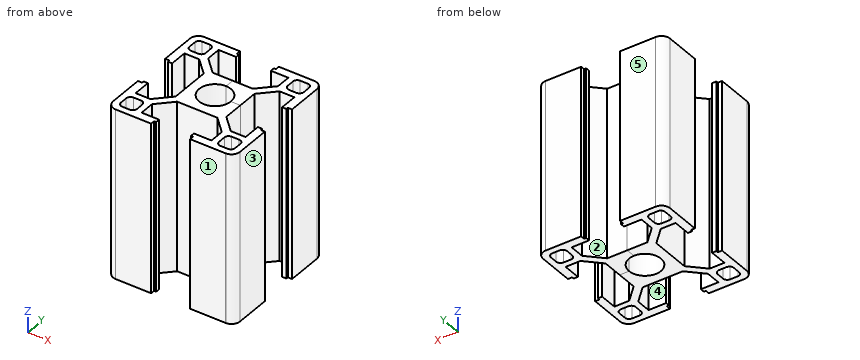
Autodesk Inventor part; units mm, degrees
ref_plane "YZ Plane" through (0, 0, 0) normal (1, 0, 0) x (0, 1, 0)
ref_plane "XZ Plane" through (0, 0, 0) normal (0, 1, 0) x (-1, 0, 0)
ref_plane "XY Plane" through (0, 0, 0) normal (0, 0, 1) x (1, 0, 0)
sketch "Sketch1" plane through (0, 0, 0) normal (0, 0, 1) x (1, 0, 0)
  line L0 (-4.1, 13) -> (-4.1, 14)
  line L1 (-4.1, 14) -> (-4.6, 14)
  line L2 (-4.6, 14) -> (-4.6, 15)
  line L3 (-4.6, 14) -> (-4.6, 15)
  line L4 (-4.6, 15) -> (-13, 15)
  arc A0 (-13, 15) -> (-15, 13) centre (-13, 13) ccw
  line L5 (-15, 13) -> (-15, 4.6)
  line L6 (-15, 13) -> (-15, 4.6)
  line L7 (-15, 4.6) -> (-14, 4.6)
  line L8 (-15, 4.6) -> (-14, 4.6)
  line L9 (-14, 4.6) -> (-14, 4.1)
  line L10 (-14, 4.6) -> (-14, 4.1)
  line L11 (-14, 4.1) -> (-13, 4.1)
  line L12 (-13, 4.1) -> (-13, 8.25)
  line L13 (-13, 8.25) -> (-9.5, 8.25)
  line L14 (-13, 8.25) -> (-9.5, 8.25)
  line L15 (-9.5, 8.25) -> (-6, 4.75)
  line L16 (-6, 4.75) -> (-6, -4.75)
  line L17 (-6, 4.75) -> (-6, -4.75)
  line L18 (-6, -4.75) -> (-9.5, -8.25)
  line L19 (-14, -4.1) -> (-13, -4.1)
  line L20 (-13, -4.1) -> (-14, -4.1)
  line L21 (-14, -4.6) -> (-14, -4.1)
  line L22 (-14, -4.1) -> (-14, -4.6)
  line L23 (-15, -4.6) -> (-14, -4.6)
  line L24 (-14, -4.6) -> (-15, -4.6)
  line L25 (-8.25, 13) -> (-4.1, 13)
  line L26 (-4.1, 13) -> (-8.25, 13)
  line L27 (-8.25, 9.5) -> (-8.25, 13)
  line L28 (-8.25, 13) -> (-8.25, 9.5)
  line L29 (-4.75, 6) -> (-8.25, 9.5)
  line L30 (-8.25, 9.5) -> (-4.75, 6)
  line L31 (4.75, 6) -> (-4.75, 6)
  line L32 (-4.75, 6) -> (4.75, 6)
  line L33 (4.75, 6) -> (8.25, 9.5)
  line L34 (8.25, 13) -> (8.25, 9.5)
  line L35 (8.25, 9.5) -> (8.25, 13)
  line L36 (8.25, 13) -> (4.1, 13)
  line L37 (4.1, 13) -> (4.1, 14)
  line L38 (4.6, 14) -> (4.1, 14)
  line L39 (4.1, 14) -> (4.6, 14)
  line L40 (4.6, 15) -> (4.6, 14)
  line L41 (4.6, 14) -> (4.6, 15)
  line L42 (4.6, 15) -> (13.08, 15)
  line L43 (15, 4.6) -> (15, 13)
  line L44 (15, 13) -> (15, 4.6)
  line L45 (14, 4.6) -> (15, 4.6)
  line L46 (15, 4.6) -> (14, 4.6)
  line L47 (14, 4.6) -> (14, 4.1)
  line L48 (13, 4.1) -> (14, 4.1)
  line L49 (14, 4.1) -> (13, 4.1)
  line L50 (13, 4.1) -> (13, 8.25)
  line L51 (9.5, 8.25) -> (13, 8.25)
  line L52 (13, 8.25) -> (9.5, 8.25)
  line L53 (6, 4.75) -> (9.5, 8.25)
  line L54 (9.5, 8.25) -> (6, 4.75)
  line L55 (6, 4.75) -> (6, -4.75)
  circle A1 centre (0, 0) radius 3.75
  line L56 (0, 0) -> (7.2487, 0)
  arc A2 (15, 13) -> (13, 15) centre (13, 13) ccw
  arc A3 (15, 13) -> (13.08, 15) centre (12.9977, 12.9994) ccw
  line L57 (-9.5, -8.25) -> (-6, -4.75)
  line L58 (-8.25, -9.5) -> (-4.75, -6)
  line L59 (-4.75, -6) -> (-8.25, -9.5)
  line L60 (-4.1, -13) -> (-4.1, -14)
  line L61 (-4.1, -14) -> (-4.6, -14)
  line L62 (-8.25, -13) -> (-4.1, -13)
  line L63 (-4.1, -13) -> (-8.25, -13)
  line L64 (-8.25, -9.5) -> (-8.25, -13)
  line L65 (-8.25, -13) -> (-8.25, -9.5)
  line L66 (-13, -8.25) -> (-9.5, -8.25)
  line L67 (-13, -4.1) -> (-13, -8.25)
  line L68 (-4.6, -14) -> (-4.6, -15)
  line L69 (-4.6, -14) -> (-4.6, -15)
  line L70 (-4.6, -15) -> (-13, -15)
  line L71 (-14, -4.6) -> (-14, -4.1)
  line L72 (-14, -4.6) -> (-14, -4.1)
  line L73 (-14, -4.1) -> (-13, -4.1)
  line L74 (-15, -4.6) -> (-14, -4.6)
  line L75 (-15, -4.6) -> (-14, -4.6)
  line L76 (-15, -13) -> (-15, -4.6)
  line L77 (-15, -13) -> (-15, -4.6)
  arc A4 (-15, -13) -> (-13, -15) centre (-13, -13) ccw
  line L78 (-13, -8.25) -> (-9.5, -8.25)
  line L79 (8.25, -13) -> (8.25, -9.5)
  line L80 (8.25, -9.5) -> (8.25, -13)
  line L81 (9.5, -8.25) -> (13, -8.25)
  line L82 (13, -8.25) -> (9.5, -8.25)
  line L83 (15, -13) -> (15, -4.6)
  line L84 (15, -4.6) -> (15, -13)
  line L85 (13, -4.1) -> (13, -8.25)
  line L86 (13, -4.1) -> (14, -4.1)
  line L87 (14, -4.1) -> (13, -4.1)
  line L88 (14, -4.6) -> (14, -4.1)
  line L89 (14, -4.6) -> (15, -4.6)
  line L90 (15, -4.6) -> (14, -4.6)
  line L91 (4.75, -6) -> (8.25, -9.5)
  line L92 (6, -4.75) -> (9.5, -8.25)
  line L93 (9.5, -8.25) -> (6, -4.75)
  arc A5 (13, -15) -> (15, -13) centre (13, -13) ccw
  arc A6 (13.08, -15) -> (15, -13) centre (12.9977, -12.9994) ccw
  line L94 (8.25, -13) -> (4.1, -13)
  line L95 (4.1, -13) -> (4.1, -14)
  line L96 (4.6, -14) -> (4.1, -14)
  line L97 (4.1, -14) -> (4.6, -14)
  line L98 (4.6, -15) -> (4.6, -14)
  line L99 (4.6, -14) -> (4.6, -15)
  line L100 (4.6, -15) -> (13.08, -15)
  line L101 (4.75, -6) -> (-4.75, -6)
  line L102 (-4.75, -6) -> (4.75, -6)
  circle A7 centre (0, 0) radius 3.75
  line L103 (-12.5, 13.5) -> (-10.7, 13.5)
  line L104 (-12.5, 13.5) -> (-10.7, 13.5)
  line L105 (-9.7, 12.5) -> (-9.7, 10.7)
  line L106 (-9.7, 12.5) -> (-9.7, 10.7)
  line L107 (-10.7, 9.7) -> (-12.5, 9.7)
  line L108 (-10.7, 9.7) -> (-12.5, 9.7)
  line L109 (-13.5, 12.5) -> (-13.5, 10.7)
  line L110 (-13.5, 10.7) -> (-13.5, 12.5)
  line L111 (-13.5, 12.5) -> (-13.5, 10.7)
  arc A8 (-12.5, 13.5) -> (-13.5, 12.5) centre (-12.5, 12.5) ccw
  arc A9 (-13.5, 10.7) -> (-12.5, 9.7) centre (-12.5, 10.7) ccw
  arc A10 (-13.5, 10.7) -> (-12.5, 9.7) centre (-12.5, 10.7) ccw
  arc A11 (-10.7, 9.7) -> (-9.7, 10.7) centre (-10.7, 10.7) ccw
  arc A12 (-9.7, 12.5) -> (-10.7, 13.5) centre (-10.7, 12.5) ccw
  arc A13 (-9.7, 12.5) -> (-10.7, 13.5) centre (-10.7, 12.5) ccw
  line L112 (0, 0) -> (0, 6.5)
  arc A14 (9.7, 10.7) -> (10.7, 9.7) centre (10.7, 10.7) ccw
  line L113 (9.7, 12.5) -> (9.7, 10.7)
  arc A15 (10.7, 13.5) -> (9.7, 12.5) centre (10.7, 12.5) ccw
  arc A16 (10.7, 13.5) -> (9.7, 12.5) centre (10.7, 12.5) ccw
  line L114 (9.7, 12.5) -> (9.7, 10.7)
  line L115 (12.5, 13.5) -> (10.7, 13.5)
  line L116 (12.5, 13.5) -> (10.7, 13.5)
  line L117 (10.7, 9.7) -> (12.5, 9.7)
  line L118 (10.7, 9.7) -> (12.5, 9.7)
  arc A17 (12.5, 9.7) -> (13.5, 10.7) centre (12.5, 10.7) ccw
  arc A18 (12.5, 9.7) -> (13.5, 10.7) centre (12.5, 10.7) ccw
  line L119 (13.5, 12.5) -> (13.5, 10.7)
  line L120 (13.5, 10.7) -> (13.5, 12.5)
  line L121 (13.5, 12.5) -> (13.5, 10.7)
  arc A19 (13.5, 12.5) -> (12.5, 13.5) centre (12.5, 12.5) ccw
  arc A20 (-13.5, -12.5) -> (-12.5, -13.5) centre (-12.5, -12.5) ccw
  line L122 (-9.7, -12.5) -> (-9.7, -10.7)
  line L123 (-9.7, -12.5) -> (-9.7, -10.7)
  line L124 (-10.7, -9.7) -> (-12.5, -9.7)
  line L125 (-10.7, -9.7) -> (-12.5, -9.7)
  line L126 (-13.5, -12.5) -> (-13.5, -10.7)
  line L127 (-13.5, -10.7) -> (-13.5, -12.5)
  line L128 (-13.5, -12.5) -> (-13.5, -10.7)
  arc A21 (-12.5, -9.7) -> (-13.5, -10.7) centre (-12.5, -10.7) ccw
  arc A22 (-12.5, -9.7) -> (-13.5, -10.7) centre (-12.5, -10.7) ccw
  arc A23 (-9.7, -10.7) -> (-10.7, -9.7) centre (-10.7, -10.7) ccw
  line L129 (-12.5, -13.5) -> (-10.7, -13.5)
  line L130 (-12.5, -13.5) -> (-10.7, -13.5)
  arc A24 (-10.7, -13.5) -> (-9.7, -12.5) centre (-10.7, -12.5) ccw
  arc A25 (-10.7, -13.5) -> (-9.7, -12.5) centre (-10.7, -12.5) ccw
  line L131 (12.5, -13.5) -> (10.7, -13.5)
  line L132 (12.5, -13.5) -> (10.7, -13.5)
  line L133 (9.7, -12.5) -> (9.7, -10.7)
  line L134 (9.7, -12.5) -> (9.7, -10.7)
  arc A26 (9.7, -12.5) -> (10.7, -13.5) centre (10.7, -12.5) ccw
  arc A27 (9.7, -12.5) -> (10.7, -13.5) centre (10.7, -12.5) ccw
  line L135 (13.5, -10.7) -> (13.5, -12.5)
  line L136 (13.5, -12.5) -> (13.5, -10.7)
  line L137 (13.5, -12.5) -> (13.5, -10.7)
  arc A28 (12.5, -13.5) -> (13.5, -12.5) centre (12.5, -12.5) ccw
  arc A29 (13.5, -10.7) -> (12.5, -9.7) centre (12.5, -10.7) ccw
  arc A30 (13.5, -10.7) -> (12.5, -9.7) centre (12.5, -10.7) ccw
  arc A31 (10.7, -9.7) -> (9.7, -10.7) centre (10.7, -10.7) ccw
  line L138 (10.7, -9.7) -> (12.5, -9.7)
  line L139 (10.7, -9.7) -> (12.5, -9.7)
  point P0 (14.7321, -14)
  point P1 (14.7321, 14)
  point P2 (14.7321, 14)
  point P3 (14.7321, -14)
extrude "Extrusion1" add sketch "Sketch1" along normal blind 40 contours L25 L27 L29 L31 L112 A1 L56 L55 L92 L81 L85 L86 L88 L89 L83 A5 L100 L98 L96 L95 L94 L79 L91 L101 L58 L64 L62 L60 L61 L68 L70 A4 L76 L23 L21 L19 L67 L66 L18 L16 L15 L13 L12 L11 L9 L7 L5 A0 L4 L2 L1 L0 | L31 L33 L34 L36 L37 L38 L40 L42 A2 L43 L45 L47 L48 L50 L51 L53 L55 L56 A1 L112
properties part number "30x30 aluminum" material "Aluminum 6061"
Verification items for the finished model (mm, model axes). Face numbers are marked on the shaded views. A direction names the side the tool comes from. Coordinates: 2 decimals unless noted, no trailing zeros. Order: outer loops, then holes, each group sorted by start corner. A loop starts at its lowest first (then second) coordinate and runs counter-clockwise, first axis right, second up. Notation, with made-up numbers: M 35,26 L 69,26 A24 ccw 69,41 Z; hole C -27.75,78.25 d11. An arc over 180 degrees is marked long. Return JSON: item names as keys, results as strings.
1) Thickness scan on L1, parallel to X at y = 12.5, z = 28; L2, parallel to Y at x = 4.75, z = 24; L3, parallel to Y at x = -6.5, z = 7. Record the ranges inside material, lowest first. Write a range as [from, to].
Answer list:
{"L1": "[-15, -13.5], [-9.7, -8.25], [8.25, 9.7], [13.5, 15]", "L2": "[-15, -13], [-6, 6], [13, 15]", "L3": "[-15, -13], [-7.75, -5.25], [5.25, 7.75], [13, 15]"}
2) Access from +Z, -Z, +X, -X, +Y, -Y to the whole of each face (thin tool, end or side, straight path). Record for the marked faces 4 and 5.
Answer list:
{"face 4": "+Z, -Z", "face 5": "+Z, -Z, +X, -X, +Y"}
3) Release check for a two-part mould opening along Y. For the marked faces 1, 2 and 3 record: +Y half, -Y half, draft (parallel to the pull), parting line (faces both ways), or undercut.
Answer list:
{"face 1": "-Y half", "face 2": "undercut", "face 3": "draft"}
4) Cross-section at A-A, the plane x = 7. Record the boundary of the cut face in (y, z), and give its area (3 significant figures).
Answer list:
{"outline": "M -15,0 L -13,0 L -13,40 L -15,40 Z; M -8.25,0 L -5.75,0 L -5.75,40 L -8.25,40 Z; M 5.75,0 L 8.25,0 L 8.25,40 L 5.75,40 Z; M 13,0 L 15,0 L 15,40 L 13,40 Z", "area": "360 mm2"}
5) Cross-section at B-B, the plane y = -7.75. Record the boundary of the cut face in (x, z).
Answer list:
{"outline": "M -15,0 L -13,0 L -13,40 L -15,40 Z; M -9,0 L -6.5,0 L -6.5,40 L -9,40 Z; M 6.5,0 L 9,0 L 9,40 L 6.5,40 Z; M 13,0 L 15,0 L 15,40 L 13,40 Z"}
6) Cross-section at C-C, the plane z = 9. Count the separate pieces of the cut face and the enclosed holes in it, and give its area (3 significant figures).
Answer list:
{"separate pieces": "1", "enclosed holes": "5", "area": "315 mm2"}
7) Gauge pin test, flat ends, axial feed: pin 1 (6 mm diameter, centred on x = 1, z = 29.5, fed in from -Y); pin 2 (0.5 mm diameter, centred on x = -14.5, z = 25.5, fed in from +Y); pin 3 (0.8 mm diameter, centred on y = -13.5, z = 21.5, fed in from +X). Record the tip position at first contact, or that the pin passes through.
Answer list:
{"pin 1": "y = -6", "pin 2": "y = 14.56", "pin 3": "x = 15"}
